from build123d import *

# Parameters (mm, degrees)
SKETCH1_W           = 50
SKETCH1_H           = 25.18
BOSS_EXTRUDE1_DEPTH = 20
SKETCH2_W           = 44
SKETCH2_H           = 19.18
CUT_EXTRUDE1_DEPTH  = 17
CUT_EXTRUDE2_DEPTH  = 3
SKETCH5_R           = 2
SKETCH5_W           = 0.418499832
SKETCH5_H           = 1.291345909
SKETCH5_W_2         = 10
SKETCH5_H_2         = 6
SKETCH5_H_3         = 4
CUT_EXTRUDE3_DEPTH  = 3
FILLET1_R           = 3
SKETCH7_W           = 6
SKETCH7_H           = 6
SKETCH7_R           = 1.5
BOSS_EXTRUDE2_DEPTH = 16
BOSS_EXTRUDE3_DEPTH = 30


with BuildPart() as part:
    # Sketch1 → Boss-Extrude1 (new body)
    with BuildSketch(Plane(origin=(0, 0, 0), x_dir=(1, 0, 0), z_dir=(0, 1, 0))):
        Rectangle(SKETCH1_W, SKETCH1_H)
    extrude(amount=BOSS_EXTRUDE1_DEPTH)

    # Sketch2 → Cut-Extrude1 (cut)
    with BuildSketch(Plane(origin=(0, 20, 0), x_dir=(1, 0, 0), z_dir=(0, 1, 0))):
        Rectangle(SKETCH2_W, SKETCH2_H)
    extrude(amount=-CUT_EXTRUDE1_DEPTH, mode=Mode.SUBTRACT)

    # Sketch4 → Cut-Extrude2 (cut)
    with BuildSketch(Plane.XY.offset(12.59)):
        with BuildLine():
            Line((-17, 20), (17, 20))
            ThreePointArc((17, 20), (0, 3), (-17, 20))
        make_face()
    extrude(amount=-CUT_EXTRUDE2_DEPTH, mode=Mode.SUBTRACT)

    # Sketch5 → Cut-Extrude3 (cut)
    with BuildSketch(Plane(origin=(0, 0, -12.59), x_dir=(-1, 0, 0), z_dir=(0, 0, -1))):
        with Locations((0.05, 15.95)):
            Circle(SKETCH5_R)
        with Locations((-49.48479677, 33.064984315)):
            Rectangle(SKETCH5_W, SKETCH5_H)
        with Locations((-17, 17)):
            Rectangle(SKETCH5_W_2, SKETCH5_H_2)
        with Locations((11.49, 10.56)):
            Rectangle(SKETCH5_W_2, SKETCH5_H_3)
    extrude(amount=-CUT_EXTRUDE3_DEPTH, mode=Mode.SUBTRACT)

    # Fillet1
    fillet1_edges = [part.edges().sort_by_distance(p)[0] for p in [
        (22, 3, 0),
        (-22, 3, 0),
    ]]
    fillet(fillet1_edges, radius=FILLET1_R)

    # Sketch7 → Boss-Extrude2 (add)
    with BuildSketch(Plane.XZ):
        with Locations((-28, 0)):
            Rectangle(SKETCH7_W, SKETCH7_H)
        with Locations((-28, 0)):
            Circle(SKETCH7_R, mode=Mode.SUBTRACT)
        with Locations((28, 0)):
            Rectangle(SKETCH7_W, SKETCH7_H)
        with Locations((28, 0)):
            Circle(SKETCH7_R, mode=Mode.SUBTRACT)
    extrude(amount=-BOSS_EXTRUDE2_DEPTH)

    # Sketch8 → Boss-Extrude3 (add)
    with BuildSketch(Plane.XZ):
        Polygon((-25, -6), (-34, -6), (-34, 6), (-25, 6), (-25, 3), (-31, 3), (-31, -3), (-25, -3), align=None)
        Polygon((25, 3), (25, 6), (34, 6), (34, -6), (25, -6), (25, -3), (31, -3), (31, 3), align=None)
    extrude(amount=-BOSS_EXTRUDE3_DEPTH)


solid = part.part
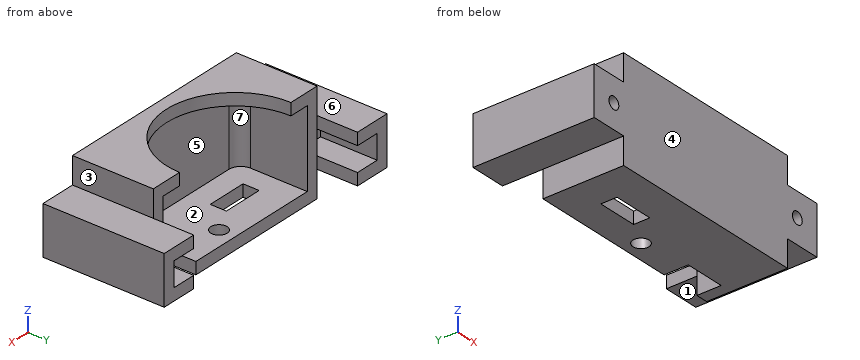
Verification items for the finished model (mm, model axes). Face numbers are marked on the shaded views. A direction names the side the tool comes from. Give positions to 0.01 mm unless a question says otherwise; leave off trailing zeros. Write each loop counter-clockwise with the first axis right and the second up, starting at its lowest first coordinate (ties: lowest second). Pieces come first, ordered by that corner, then holes. Notation, with made-up numbers: M 12,9 L 27,9 A20 cw 27,20 Z; hole C 13,14 d3. An arc over 180 degrees is marked long. Put each result on its own line as item: value. Start each with the question number.
1. Section check C-C (z = 8.5). Record the cut outline in (x, y), and give its area (3 significant figures).
2. Scan lines: line 1 along Z through (x, y) = (-19.5, 11.25); line 2 along Z through (x, y) = (28, 12); line 3 along X through (y, z) = (17.25, -8). Record each from-to range of solid material in increasing order. Write a range as [from, to].
3. Section check A-A (y = 9.25). Record the cut outline in (x, z), and give its area (3 significant figures).
4. Set-up check for the marked faces 1, 2 and 3: record each of +Z, -Z, +X, -X, +Y, -Y from which the full face is reachable in a straight line by a thin tool's end or side.
5. Go/stop test with flat-tipped pins: pin 1 Ø9.5 at (x, z) = (2, -1.5) entering from +Y; pin 2 Ø2.5 at (x, z) = (-12.5, -10.5) entering from +Y; pin 3 Ø10 at (x, y) = (31.5, 16) entering from -Z; pin 4 Ø2.5 at (x, z) = (-28, 0) entering from +Y. Record where each tip stops, or that it passes through.
6. Section check D-D (y = 17). Give the number of separate pieces and of enclosed holes in the cut face, and give its area (3 significant figures).
7. Draft check along Z on the marked faces 4, 5, 6 and 7. Enter one of: +Z half, -Z half, draft (parallel to the pull), parting line (faces both ways), or undercut.
8. Section check B-B (x = 28.5). Record the cut outline in (y, z), and give its area (3 significant figures).
Answer list:
1. outline: M -25,0 L 25,0 L 25,20 L 22,20 L 22,6 A3 cw 19,3 L -19,3 A3 cw -22,6 L -22,20 L -25,20 Z
1. area: 256 mm2
2. line 1: [-12.59, -9.59], [9.59, 12.59]
2. line 2: [-6, -1.5], [1.5, 6]
2. line 3: [-25, -22], [22, 25]
3. outline: M -34,-6 L -25,-6 L -25,-12.59 L -16.49,-12.59 L -16.49,-9.59 L -22,-9.59 L -22,9.59 L -13.17,9.59 L -13.17,12.59 L -25,12.59 L -25,6 L -34,6 Z; M -6.49,-12.59 L 25,-12.59 L 25,-6 L 34,-6 L 34,6 L 25,6 L 25,12.59 L 13.17,12.59 L 13.17,9.59 L 22,9.59 L 22,-9.59 L -6.49,-9.59 Z; hole C -28,0 d3; hole C 28,0 d3
3. area: 508 mm2
4. face 1: -Z, +X, +Y, -Y
4. face 2: +Y
4. face 3: +Z, +X, +Y, -Y
5. pin 1: y = 3
5. pin 2: y = 20
5. pin 3: z = -6
5. pin 4: through
6. separate pieces: 3
6. enclosed holes: 2
6. area: 418 mm2
7. face 4: draft
7. face 5: undercut
7. face 6: +Z half
7. face 7: undercut
8. outline: M 0,-6 L 30,-6 L 30,-3 L 16,-3 L 16,-1.41 L 0,-1.41 Z; M 0,1.41 L 16,1.41 L 16,3 L 30,3 L 30,6 L 0,6 Z
8. area: 231 mm2
